Could you check a few things on this model? Use its own coordinates, in mm. Face numbers are marked on the shaded views. A direction names the side the tool comes from. Give positions to 0.01 mm unless a question says otherwise; leave off trailing zeros. Loops run counter-clockwise (first coordinate to the right, second up) from the corner with the lowest first, then second, coordinate; pieces in that order, holes last. Notation, with made-up numbers: (38.5, -15.75) - (58.5, -15.75) arc R27 ccw to (58.5, 23.25) - close; hole circle Ø7 at (-34.5, 71.5). An arc over 180 degrees is marked (long way). One line per item, written item: value. Start each with the question number.
Q1. If we mould it in two halves opening along Z, with no side actions, what happens to the marked faces 1, 2, 3 and 4? For each: released by +Z, released by -Z, zero draft, split by the parting line, or undercut.
Q2. For the marked faces 5, 6 and 7, which set-ups out of +Z, -Z, +X, -X, +Y, -Y let a thin tool reach every point of the face, with its end or its side?
Q3. I'm going to push flat-ended pins straight in: P1, Ø1.5, axis at x = 16, y = 1, coming from the +Z side; P2, Ø2, axis at x = 4.5, z = -6.5, coming from the -Y side; P3, Ø3.5, axis at x = -4, z = 10, coming from the +Y side; P4, Ø1.3, axis at y = 1.5, z = -10, coming from the +X side. Where does each tip first touch, or does it pass through?
Q4. I want a section at A-A (x = -4). Please give me the cut outline in (y, z), then the cut area to 3 significant figures.
Q5. I want a section at C-C (y = 3.35). Please give me the cut outline in (x, z).
Q6. If I drill on line 1 (Z direction, x = -4, y = 2.3); line 2 (X direction, y = 3.3, z = 10); line 3 (Z direction, x = -3.5, y = 2.4), over which ranges is the centre line in solid material (lowest first)? Write a range as from..to.
Q7. I want a section at B-B (z = 0). Please give me the cut outline in (x, y).
Q8. I want a section at D-D (x = 14.5). Please give me the cut outline in (y, z).
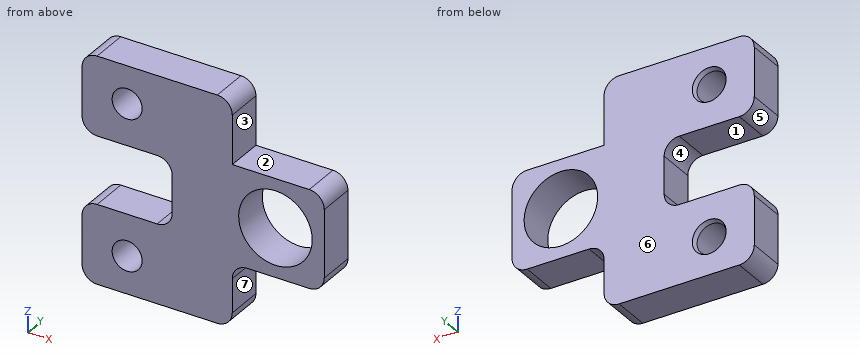
```python
from build123d import *

# Parameters (mm, degrees)
SKETCH1_R                         = 4.9
BOSS_EXTRUDE1_DEPTH               = 5
FILLET1_R                         = 2
F_4_0_4_DIAMETER_HOLE1_AT_2_COUNT = 2
F_4_0_4_DIAMETER_HOLE1_AT_2_PITCH = 10
F_4_0_4_DIAMETER_HOLE1_AT_3_COUNT = 2
F_4_0_4_DIAMETER_HOLE1_AT_3_PITCH = 10


with BuildPart() as part:
    # Sketch1 → Boss-Extrude1 (new body)
    with BuildSketch(Plane(origin=(0, 0, 0), x_dir=(1, 0, 0), z_dir=(0, 1, 0))):
        Polygon((-10, 15), (-10, 4.5), (2, 4.5), (2, -4.5), (-10, -4.5), (-10, -15), (10, -15), (10, -6.5), (22.25, -6.5), (22.25, 6.5), (10, 6.5), (10, 15), align=None)
        with Locations(Location((15.75, 0, 0), (0, 0, 270))):
            Circle(SKETCH1_R, mode=Mode.SUBTRACT)
    extrude(amount=BOSS_EXTRUDE1_DEPTH)

    # Fillet1
    fillet1_edges = [part.edges().sort_by_distance(p)[0] for p in [
        (10, 2.5, 15),
        (-10, 2.5, 15),
        (-10, 2.5, 4.5),
        (2, 2.5, 4.5),
        (2, 2.5, -4.5),
        (-10, 2.5, -4.5),
        (-10, 2.5, -15),
        (10, 2.5, -15),
        (10, 2.5, -6.5),
        (22.25, 2.5, -6.5),
        (22.25, 2.5, 6.5),
    ]]
    fillet(fillet1_edges, radius=FILLET1_R)

    # Sketch5 → Ø4.0 (4) Diameter Hole1 (revolve, cut)
    with BuildSketch(Plane(origin=(-4, 5, 0), x_dir=(0, 0, 1), z_dir=(1, 0, 0))):
        Polygon((0, 0), (0, 5), (2, 5), (2, 0.603553391), (2.25, 0), align=None)
    f_4_0_4_diameter_hole1 = revolve(axis=Axis((-4, 11.35, 0), (0, -1, 0)), mode=Mode.SUBTRACT)

    # Ø4.0 (4) Diameter Hole1 at 2: Ø4.0 (4) Diameter Hole1 ×2
    with Locations(*[(0, 0, i * F_4_0_4_DIAMETER_HOLE1_AT_2_PITCH) for i in range(1, F_4_0_4_DIAMETER_HOLE1_AT_2_COUNT)]):
        add(f_4_0_4_diameter_hole1, mode=Mode.SUBTRACT)

    # Ø4.0 (4) Diameter Hole1 at 3: Ø4.0 (4) Diameter Hole1 ×2
    with Locations(*[(0, 0, -i * F_4_0_4_DIAMETER_HOLE1_AT_3_PITCH) for i in range(1, F_4_0_4_DIAMETER_HOLE1_AT_3_COUNT)]):
        add(f_4_0_4_diameter_hole1, mode=Mode.SUBTRACT)


solid = part.part
```
Worked answers:
1. face 1: undercut
1. face 2: released by +Z
1. face 3: zero draft
1. face 4: undercut
2. face 5: -X, +Y, -Y
2. face 6: +Z, -Z, +X, -X, +Y
2. face 7: -Z, +X, +Y, -Y
3. P1: stops at z = 6.5
3. P2: stops at y = 0
3. P3: passes through
3. P4: stops at x = 10
4. outline: (0, -15) - (5, -15) - (5, -12.25) - (4.4, -12) - (0, -12) - close; (0, -8) - (4.4, -8) - (5, -7.75) - (5, -4.5) - (0, -4.5) - close; (0, 4.5) - (5, 4.5) - (5, 7.75) - (4.4, 8) - (0, 8) - close; (0, 12) - (4.4, 12) - (5, 12.25) - (5, 15) - (0, 15) - close
4. area: 64.7 mm²
5. outline: (-10, -13) arc R2 ccw to (-8, -15) - (8, -15) arc R2 ccw to (10, -13) - (10, -8.5) arc R2 cw to (12, -6.5) - (20.25, -6.5) arc R2 ccw to (22.25, -4.5) - (22.25, 4.5) arc R2 ccw to (20.25, 6.5) - (10, 6.5) - (10, 13) arc R2 ccw to (8, 15) - (-8, 15) arc R2 ccw to (-10, 13) - (-10, 6.5) arc R2 ccw to (-8, 4.5) - (0, 4.5) arc R2 cw to (2, 2.5) - (2, -2.5) arc R2 cw to (0, -4.5) - (-8, -4.5) arc R2 ccw to (-10, -6.5) - close; hole circle Ø4 at (-4, -10); hole circle Ø4 at (-4, 10); hole circle Ø9.8 at (15.75, 0)
6. line 1: z = -15..-12, -8..-4.5, 4.5..8, 12..15
6. line 2: x = -10..-6, -2..10
6. line 3: z = -15..-11.94, -8.06..-4.5, 4.5..8.06, 11.94..15
7. outline: (2, 0) - (10.85, 0) - (10.85, 5) - (2, 5) - close; (20.65, 0) - (22.25, 0) - (22.25, 5) - (20.65, 5) - close
8. outline: (0, -6.5) - (5, -6.5) - (5, -4.74) - (0, -4.74) - close; (0, 4.74) - (5, 4.74) - (5, 6.5) - (0, 6.5) - close
